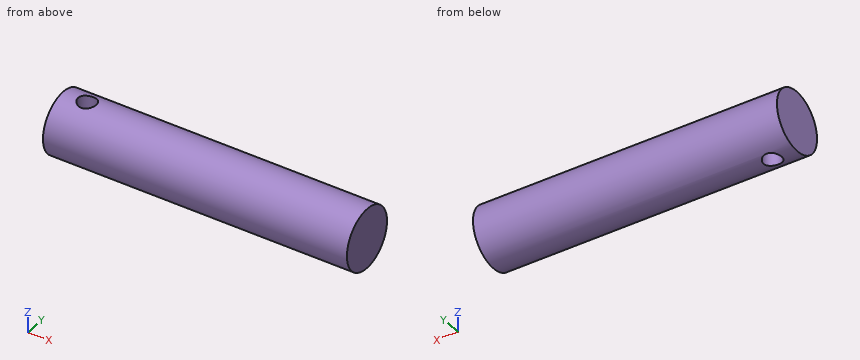
from build123d import *

# Parameters (mm, degrees)
SKIZZE1_W                                   = 100
SKIZZE1_H                                   = 10
SCHNITT_LINEAR_AUSTRAGEN1_REACH             = 12
SKIZZE2_R                                   = 3
SCHNITT_LINEAR_AUSTRAGEN1_DIRECTION_2_REACH = 12


with BuildPart() as part:
    # Skizze1 → Rotation1 (revolve)
    with BuildSketch(Plane.XY):
        with Locations((50, 5)):
            Rectangle(SKIZZE1_W, SKIZZE1_H)
    revolve(axis=Axis((0, 0, 0), (1, 0, 0)))

    # Skizze2 → Schnitt-Linear austragen1 (cut, up to next)
    with BuildSketch(Plane.XY, mode=Mode.PRIVATE) as schnitt_linear_austragen1_sk1:
        with Locations((8, 0)):
            Circle(SKIZZE2_R)
    schnitt_linear_austragen1_tool1 = extrude(schnitt_linear_austragen1_sk1.sketch, amount=-SCHNITT_LINEAR_AUSTRAGEN1_REACH, mode=Mode.PRIVATE) & part.part
    add(schnitt_linear_austragen1_tool1.solids().sort_by_distance((8, 0, 0))[0], mode=Mode.SUBTRACT)

    # Skizze2 → Schnitt-Linear austragen1 direction 2 (cut, up to next)
    with BuildSketch(Plane.XY, mode=Mode.PRIVATE) as schnitt_linear_austragen1_direction_2_sk1:
        with Locations((8, 0)):
            Circle(SKIZZE2_R)
    schnitt_linear_austragen1_direction_2_tool1 = extrude(schnitt_linear_austragen1_direction_2_sk1.sketch, amount=SCHNITT_LINEAR_AUSTRAGEN1_DIRECTION_2_REACH, mode=Mode.PRIVATE) & part.part
    add(schnitt_linear_austragen1_direction_2_tool1.solids().sort_by_distance((8, 0, 0))[0], mode=Mode.SUBTRACT)


solid = part.part
Check sheet for the modelled part. Datum: model origin and axes. Units: mm. Give positions to 0.01 mm unless a question says otherwise; leave off trailing zeros. Order: outer loops, then holes, each group sorted by start corner. A loop starts at its lowest first (then second) coordinate and runs counter-clockwise, first axis right, second up. Notation, with made-up numbers: M 4.5,54.25 L 37.5,54.25 A18 cw 37.5,85.25 Z; hole C 22,35 d4. An arc over 180 degrees is marked long. Answer as CSV lines item,"result". Start each with the question number.
Item 1: Cross-section at B-B on x = 30.5. Enter the section's corners in (y, z).
Item 2: Gauge pin test, flat ends, axial feed: P1, Ø4, axis at x = 57, y = -5, coming from the +Z side; P2, Ø1.5, axis at x = 88, y = 5, coming from the -Z side; P3, Ø1.5, axis at x = 69.5, y = -3.5, coming from the -Z side. Record the tip position at first contact, or that the pin passes through.
Item 3: Cross-section at D-D on y = -6.25. Enter the section's corners in (x, z), plus the area to 3 significant figures.
Item 4: Cross-section at C-C on x = 8. Enter the section's corners in (y, z), plus the area to 3 significant figures.
Item 5: Thickness scan on line 1 (X direction, y = 0, z = -5.75); line 2 (X direction, y = -1.75, z = -4.5); line 3 (Y direction, x = 8, z = 2.25). Record the ranges inside material, lowest first. Write a range as [from, to].
Item 6: Cross-section at A-A on z = -1.5. Enter the section's corners in (x, y), plus the area to 3 significant figures.
Established:
1,outline,"C 0,0 d20"
2,P1,"stops at z = 9.54"
2,P2,"stops at z = -9.05"
2,P3,"stops at z = -9.61"
3,outline,"M 0,-7.81 L 100,-7.81 L 100,7.81 L 0,7.81 Z"
3,area,"1,560 mm^2"
4,outline,"M -3,-9.54 L -3,9.54 A10 ccw Z; M 3,-9.54 A10 ccw 3,9.54 Z"
4,area,"196 mm^2"
5,line 1,"x = [0, 5], [11, 100]"
5,line 2,"x = [0, 5.56], [10.44, 100]"
5,line 3,"y = [-9.74, -3], [3, 9.74]"
6,outline,"M 0,-9.89 L 100,-9.89 L 100,9.89 L 0,9.89 Z; hole C 8,0 d6"
6,area,"1,950 mm^2"
